Can you work these out from the model? Positions are in its coordinate system, mm. A direction names the side the tool comes from. Give positions to 0.01 mm unless a question says otherwise; leave off trailing zeros. Order: outer loops, then holes, each group sorted by start corner. A loop starts at its lowest first (then second) coordinate and runs counter-clockwise, first axis right, second up. Notation, with made-up numbers: (68, 2.5) - (111, 2.5) arc R35 cw to (111, 37.5) - close; hole circle Ø4 at (-3.75, 37.25). An arc over 180 degrees is marked (long way). One line per question, with ' | ' between items.
```python
from build123d import *

# Parameters (mm, degrees)
SKETCH1_R                                    = 2.8
BOSS_EXTRUDE1_DEPTH                          = 10.8
BOSS_EXTRUDE2_DEPTH                          = 40
BOSS_EXTRUDE5_START                          = 20
SKETCH1_7_R                                  = 6.3
SKETCH1_7_R_2                                = 2.8
BOSS_EXTRUDE5_DEPTH                          = 8.4
CSK_FOR_M6_COUNTERSUNK_FLAT_HEAD_SCR_2_COUNT = 2
CSK_FOR_M6_COUNTERSUNK_FLAT_HEAD_SCR_2_PITCH = 23.5


with BuildPart() as part:
    # Sketch1 → Boss-Extrude1 (new body)
    with BuildSketch(Plane(origin=(0, 0, 0), x_dir=(1, 0, 0), z_dir=(0, 1, 0))):
        with BuildLine():
            Line((-22.433809621, 0), (-6.3, 0))
            ThreePointArc((-6.3, 0), (4.454772721, -4.454772721), (0, 6.3))
            Line((0, 6.3), (-25.7, 6.3))
            Line((-25.7, 6.3), (-23.358351291, 0.618919036))
            ThreePointArc((-23.358351291, 0.618919036), (-22.990100479, 0.169012346), (-22.433809621, 0))
        make_face()
        Circle(SKETCH1_R, mode=Mode.SUBTRACT)
    extrude(amount=BOSS_EXTRUDE1_DEPTH)

    # Sketch1_3 → Boss-Extrude2 (add)
    with BuildSketch(Plane(origin=(0, 0, 0), x_dir=(1, 0, 0), z_dir=(0, 1, 0))):
        with BuildLine():
            ThreePointArc((-6.3, 0), (-4.454772721, 4.454772721), (0, 6.3))
            Line((0, 6.3), (-25.7, 6.3))
            Line((-25.7, 6.3), (-23.358351291, 0.618919036))
            ThreePointArc((-23.358351291, 0.618919036), (-22.990100479, 0.169012346), (-22.433809621, 0))
            Line((-22.433809621, 0), (-6.3, 0))
        make_face()
    extrude(amount=BOSS_EXTRUDE2_DEPTH)

    # Sketch1_7 → Boss-Extrude5 (add)
    with BuildSketch(Plane(origin=(0, 0, 0), x_dir=(1, 0, 0), z_dir=(0, 1, 0)).offset(BOSS_EXTRUDE5_START)):
        Circle(SKETCH1_7_R)
        Circle(SKETCH1_7_R_2, mode=Mode.SUBTRACT)
    extrude(amount=BOSS_EXTRUDE5_DEPTH)

    # Sketch3 → CSK for M6 Countersunk Flat Head Screw1 (revolve, cut)
    with BuildSketch(Plane(origin=(-15.7, 31.75, 0), x_dir=(0, -1, 0), z_dir=(1, 0, 0))):
        Polygon((0, 0), (0, 6.3), (3.2, 6.3), (3.2, 3.6), (6.3, 0.5), (6.3, 0), align=None)
    csk_for_m6_countersunk_flat_head_screw1 = revolve(axis=Axis((-15.7, 31.75, 6.35), (0, 0, -1)), mode=Mode.SUBTRACT)

    # CSK for M6 Countersunk Flat Head Scr 2: CSK for M6 Countersunk Flat Head Screw1 ×2
    with Locations(*[(0, -i * CSK_FOR_M6_COUNTERSUNK_FLAT_HEAD_SCR_2_PITCH, 0) for i in range(1, CSK_FOR_M6_COUNTERSUNK_FLAT_HEAD_SCR_2_COUNT)]):
        add(csk_for_m6_countersunk_flat_head_screw1, mode=Mode.SUBTRACT)


solid = part.part
```
(1) If we mould it in two halves opening along X, with no side actions, what happens to faces 6 (the face through (-24.546, 19.72, -3.499)), 7 (the face through (-14, 20, 0)), 8 (the face through (-15.841, 34.947, -4.931))? For each: released by +X, released by -X, zero draft, split by the parting line, or undercut.
Answer below:
face 6: released by -X | face 7: zero draft | face 8: undercut
(2) Imagine slicing it at A-A (y = 8.25). List the corners of the cut face in (x, z) for me, and give its area (3 significant figures).
Answer below:
outline: (-25.7, -6.3) - (-18.9, -6.3) - (-18.9, -3.6) - (-22, -0.5) - (-22, 0) - (-22.43, 0) arc R1 ccw to (-23.36, -0.62) - close; (-12.5, -6.3) - (0, -6.3) arc R6.3 ccw (long way) to (-6.3, 0) - (-9.4, 0) - (-9.4, -0.5) - (-12.5, -3.6) - close; hole circle Ø5.6 at (0, 0) | area: 170 mm^2
(3) If I drill on line 1 (Y direction, x = -15.7, z = -4.7); line 2 (Y direction, x = -15.7, z = -0.15); line 3 (X direction, y = 8.25, z = -0.1), over which ranges is the centre line in solid material (lowest first)?
Answer below:
line 1: 0 to 5.05, 11.45 to 28.55, 34.95 to 40 | line 2: 0 to 1.95, 14.55 to 25.45, 38.05 to 40 | line 3: -22.87 to -22, -9.4 to -2.8, 2.8 to 6.3
(4) Imagine slicing it at C-C (x = -15.7). List the corners of the cut face in (y, z) for me.
Answer below:
outline: (0, -6.3) - (5.05, -6.3) - (5.05, -3.6) - (1.95, -0.5) - (1.95, 0) - (0, 0) - close; (11.45, -6.3) - (28.55, -6.3) - (28.55, -3.6) - (25.45, -0.5) - (25.45, 0) - (14.55, 0) - (14.55, -0.5) - (11.45, -3.6) - close; (34.95, -6.3) - (40, -6.3) - (40, 0) - (38.05, 0) - (38.05, -0.5) - (34.95, -3.6) - close
(5) Will these pins go through, and if not, where does the flat tip stop? pin 1 (4 mm diameter, centred on x = -3, z = 1.5, fed in from +Y); pin 2 (17.5 mm diameter, centred on x = -14.5, y = 24.5, fed in from +Z); pin 3 (8 mm diameter, centred on x = -13, y = 34.5, fed in from +Z).
Answer below:
pin 1: y = 28.4 | pin 2: z = 2.57 | pin 3: z = 0
(6) On a 3-axis mill with a long thin cutter (end or side, diameter ignored), from which of +Z, -Z, +X, -X, +Y, -Y can I reach the whole of each face in a straight line? I mean faces 1 (the face through (-6, 0, -1)), 2 (the face through (3, 20, 1)), 3 (the face through (-9.55, 9.62, -0.25)), 4 (the face through (-4.5, 34.12, -4.41)), 5 (the face through (4.305, 5.324, 4.599)). Say none if no direction works.
Answer below:
face 1: +Z, -Z, +X, -X, -Y | face 2: +Z, +X | face 3: +Z | face 4: +Z, +X, +Y | face 5: +Y, -Y
(7) Imagine slicing it at D-D (z = 3.25). List the corners of the cut face in (x, y) for me.
Answer below:
outline: (-5.4, 0) - (5.4, 0) - (5.4, 10.8) - (-5.4, 10.8) - close; (-5.4, 20) - (5.4, 20) - (5.4, 28.4) - (-5.4, 28.4) - close
(8) Imagine slicing it at B-B (y = 31.75). List the corners of the cut face in (x, z) for me, and give its area (3 significant figures).
Answer below:
outline: (-25.7, -6.3) - (-18.9, -6.3) - (-18.9, -3.6) - (-22, -0.5) - (-22, 0) - (-22.43, 0) arc R1 ccw to (-23.36, -0.62) - close; (-12.5, -6.3) - (0, -6.3) arc R6.3 cw to (-6.3, 0) - (-9.4, 0) - (-9.4, -0.5) - (-12.5, -3.6) - close | area: 69.4 mm^2
